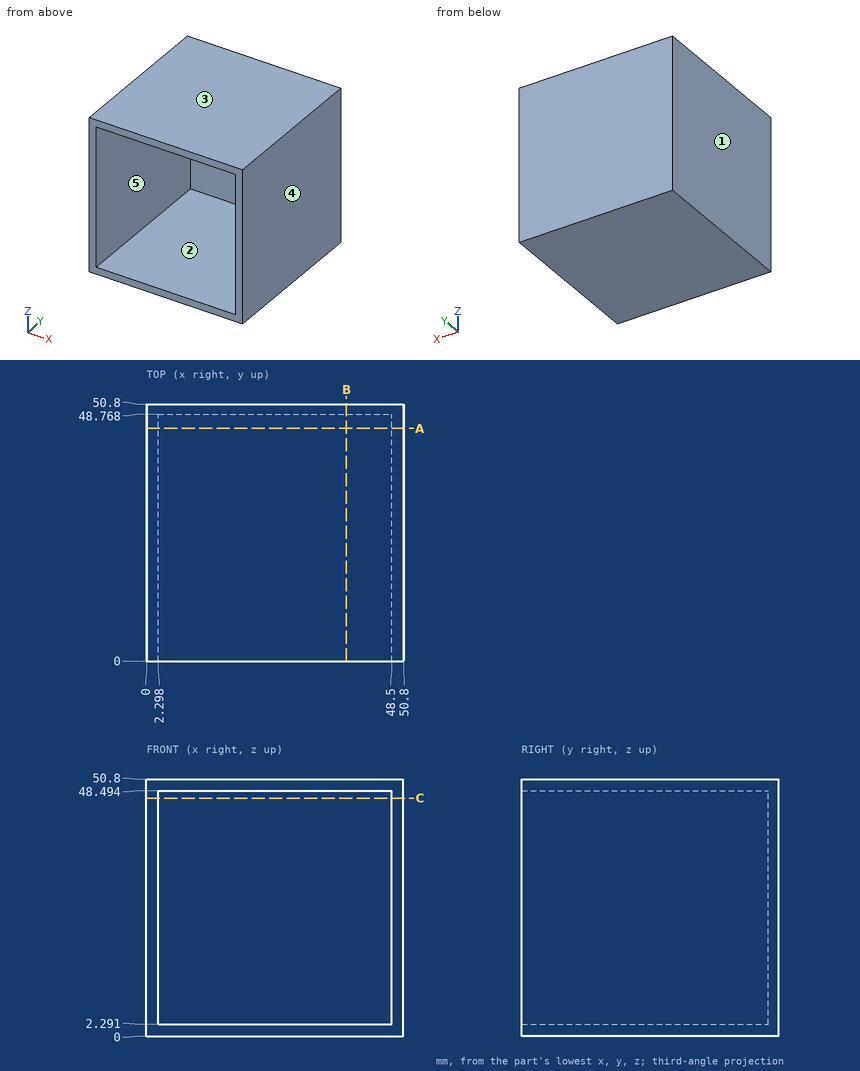
Part print with two shaded views. Sizes in mm from the minimum x, y, z corner. A direction names the side the tool comes from. Round coordinates to 2 decimals unless told otherwise and drop trailing zeros. Order: outer loops, then holes, each group sorted by start corner. A loop starts at its lowest first (then second) coordinate and runs counter-clockwise, first axis right, second up.
(1) Band-saw the part on C-C (z = 47). List the corners of the cut face in (x, y).
(2) 3-axis set-ups, long thin cutter, end or side, ignore diameter. For the marked faces 4 and 5: which of +Z, -Z, +X, -X, +Y, -Y reach the whole face in a straight line?
(3) Band-saw the part on A-A (y = 46). List the corners of the cut face in (x, z) (1 decimal).
(4) Drill centre lines: line 1 (X direction, y = 33, z = 19.5); line 2 (Y direction, x = 18.5, z = 13.5). Where is each one in solid material? Low to high.
(5) Pull direction X, two halves, no side cores. Call the marked faces 1, 2 and 3: released by +X, released by -X, zero draft, split by the parting line, or undercut.
(6) Band-saw the part on B-B (x = 39.5). List the corners of the cut face in (y, z) (1 decimal).
(7) Pin check, flat tip, straight feed: pin 1 (12 mm diameter, centred on x = 26, z = 40.5, fed in from -Y). Stop position of the tip, or through.
Verdict:
1. outline: (0, 0) - (2.3, 0) - (2.3, 48.77) - (48.5, 48.77) - (48.5, 0) - (50.8, 0) - (50.8, 50.8) - (0, 50.8) - close
2. face 4: +Z, -Z, +X, +Y, -Y
2. face 5: -Y
3. outline: (0, 0) - (50.8, 0) - (50.8, 50.8) - (0, 50.8) - close; hole (2.3, 2.3) - (48.5, 2.3) - (48.5, 48.5) - (2.3, 48.5) - close
4. line 1: x = 0 to 2.3, 48.5 to 50.8
4. line 2: y = 48.77 to 50.8
5. face 1: released by -X
5. face 2: undercut
5. face 3: zero draft
6. outline: (0, 0) - (50.8, 0) - (50.8, 50.8) - (0, 50.8) - (0, 48.5) - (48.8, 48.5) - (48.8, 2.3) - (0, 2.3) - close
7. pin 1: stops at y = 48.77
